Here's how the part is built. I have some questions about the finished solid (model axes, mm). Face numbers are marked on the shaded views. A direction names the side the tool comes from. Round coordinates to 2 decimals unless told otherwise and drop trailing zeros. Loops run counter-clockwise (first coordinate to the right, second up) from the corner with the lowest first, then second, coordinate; pieces in that order, holes last. Notation, with made-up numbers: M 19,74.5 L 73,74.5 A25 cw 73,105.5 Z; hole C -21.75,17 d10. An arc over 180 degrees is marked long. Use a Markdown table: item, result.
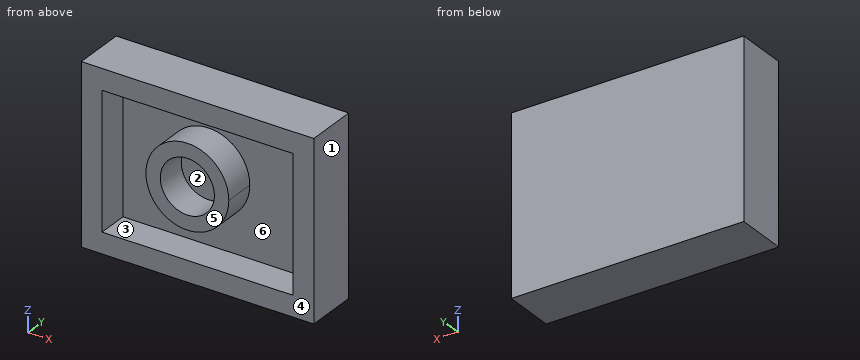
```python
from build123d import *

# Parameters (mm, degrees)
F0_W     = 111.855097
F0_H     = 85.019909
F1_DEPTH = 25
F2_T     = -10
F3_R     = 13.018473
F4_DEPTH = 25


with BuildPart() as f1:
    # F0 (on Front) → F1 (new body)
    with BuildSketch(Plane.XZ):
        with Locations((4.890524, -1.253982)):
            Rectangle(F0_W, F0_H)
    extrude(amount=F1_DEPTH)

    # F2
    f2_openings = [f1.faces().sort_by_distance(p)[0] for p in [
        (4.890524, -25, -1.253981),
    ]]
    offset(amount=F2_T, openings=f2_openings)

    # F3 (on Front) → F4 (join)
    with BuildSketch(Plane.XZ):
        with BuildLine():
            ThreePointArc((6.744158, -18.764725), (16.310675, -11.469981), (19.939874, 0))
            ThreePointArc((19.939874, 0), (-11.469981, 16.310675), (-6.744158, -18.764725))
            ThreePointArc((-6.744158, -18.764725), (0, -19.939874), (6.744158, -18.764725))
        make_face()
        Circle(F3_R, mode=Mode.SUBTRACT)
    extrude(amount=F4_DEPTH)


solid = f1.part
```
Q1. Will this pin go through, and if not, where does the flat tip stop? P1, Ø1.5, axis at x = 3, z = 25, coming from the -Y side.
Return value:
| item | result |
|---|---|
| P1 | stops at y = -10 |
Q2. Imagine slicing it at A-A, the plane y = -19.5. Please give me the cut outline in (x, z).
Return value:
| item | result |
|---|---|
| outline | M -51.04,-43.76 L 60.82,-43.76 L 60.82,41.26 L -51.04,41.26 Z; M -6.74,-18.76 A19.94 ccw 6.74,-18.76 A19.94 ccw 19.94,0 A19.94 ccw long Z; hole M -41.04,-33.76 L 50.82,-33.76 L 50.82,31.26 L -41.04,31.26 Z; hole C 0,0 d26.04 |
Q3. We'd pull the mould along X, two halves only. Please class the marked faces 1, 2, 3 and 4: pulls with the +X half, pulls with the -X half, needs draft (parallel to the pull), parting line crosses it, or undercut.
Return value:
| item | result |
|---|---|
| face 1 | pulls with the +X half |
| face 2 | undercut |
| face 3 | undercut |
| face 4 | needs draft |
Q4. For the marked faces 5 and 6, which set-ups out of +Z, -Z, +X, -X, +Y, -Y let a thin tool reach every point of the face, with its end or its side?
Return value:
| item | result |
|---|---|
| face 5 | +Z, -Z, +X, -X, -Y |
| face 6 | -Y |
Q5. Imagine slicing it at D-D, the plane x = -35. Please give me the cut outline in (y, z).
Return value:
| item | result |
|---|---|
| outline | M -25,-43.76 L 0,-43.76 L 0,41.26 L -25,41.26 L -25,31.26 L -10,31.26 L -10,-33.76 L -25,-33.76 Z |
Q6. I need wall thicknesses on line 1 (Z direction, x = 0, y = -19.25); line 2 (X direction, y = -21.25, z = 9.5); line 3 (Z direction, x = -31.5, y = -17). Which ranges of each line are inside material? Lowest first, please. Write a range as from..to.
Return value:
| item | result |
|---|---|
| line 1 | z = -43.76..-33.76, -19.94..-13.02, 13.02..19.94, 31.26..41.26 |
| line 2 | x = -51.04..-41.04, -17.53..-8.9, 8.9..17.53, 50.82..60.82 |
| line 3 | z = -43.76..-33.76, 31.26..41.26 |
Q7. Imagine slicing it at B-B, the plane x = 0. Please give me the cut outline in (y, z).
Return value:
| item | result |
|---|---|
| outline | M -25,-43.76 L 0,-43.76 L 0,41.26 L -25,41.26 L -25,31.26 L -10,31.26 L -10,19.94 L -25,19.94 L -25,13.02 L -10,13.02 L -10,-13.02 L -25,-13.02 L -25,-19.94 L -10,-19.94 L -10,-33.76 L -25,-33.76 Z |
Q8. Imagine slicing it at C-C, the plane z = 22. Please give me the cut outline in (x, y).
Return value:
| item | result |
|---|---|
| outline | M -51.04,-25 L -41.04,-25 L -41.04,-10 L 50.82,-10 L 50.82,-25 L 60.82,-25 L 60.82,0 L -51.04,0 Z |
